Model file for the job. Use its own axes, mm. A direction names the side the tool comes from. Round coordinates to 2 decimals unless told otherwise and drop trailing zeros. Loops run counter-clockwise (first coordinate to the right, second up) from the corner with the lowest first, then second, coordinate; pieces in that order, holes last. Notation, with made-up numbers: (21.25, -7) - (32.25, -7) arc R20 ccw to (32.25, 8) - close; hole circle Ø8 at (-30.5, 56.25). An arc over 180 degrees is marked (long way). Answer as a JSON object with one key per item and string values.
from build123d import *

# Parameters (mm, degrees)
BOX054_W          = 2
BOX054_H          = 2
BOX054_DEPTH      = 2
BOX051_W          = 47.5
BOX051_H          = 17.2
BOX051_DEPTH      = 27
BOX050_W          = 47.5
BOX050_H          = 18.7
BOX050_DEPTH      = 30
BOX053_W          = 10
BOX053_H          = 11.7
BOX053_DEPTH      = 6.2
FILLET001_R       = 3.05
CYLINDER038_R     = 1.7
CYLINDER038_DEPTH = 10
CYLINDER037_R     = 1.7
CYLINDER037_DEPTH = 10
CYLINDER036_R     = 1.7
CYLINDER036_DEPTH = 10
CYLINDER035_R     = 1.7
CYLINDER035_DEPTH = 10
BOX024_W          = 10
BOX024_H          = 10
BOX024_DEPTH      = 10
BOX025_W          = 10
BOX025_H          = 10
BOX025_DEPTH      = 10
CYLINDER023_R     = 4.3
CYLINDER023_DEPTH = 5
CYLINDER019_R     = 1.2
CYLINDER019_DEPTH = 10
BOX013_W          = 4.5
BOX013_H          = 4.5
BOX013_DEPTH      = 10
BOX012_W          = 7.5
BOX012_H          = 7.5
BOX012_DEPTH      = 10
CYLINDER020_R     = 1.2
CYLINDER020_DEPTH = 10
BOX015_W          = 4.5
BOX015_H          = 4.5
BOX015_DEPTH      = 10
BOX014_W          = 7.5
BOX014_H          = 7.5
BOX014_DEPTH      = 10
CYLINDER021_R     = 1.2
CYLINDER021_DEPTH = 10
BOX017_W          = 4.5
BOX017_H          = 4.5
BOX017_DEPTH      = 10
BOX016_W          = 7.5
BOX016_H          = 7.5
BOX016_DEPTH      = 10
CYLINDER022_R     = 1.2
CYLINDER022_DEPTH = 10
BOX019_W          = 4.5
BOX019_H          = 4.5
BOX019_DEPTH      = 10
BOX018_W          = 7.5
BOX018_H          = 7.5
BOX018_DEPTH      = 10
BOX022_W          = 4.5
BOX022_H          = 4.5
BOX022_DEPTH      = 10
BOX021_W          = 4.5
BOX021_H          = 4.5
BOX021_DEPTH      = 10
BOX023_W          = 4.5
BOX023_H          = 4.5
BOX023_DEPTH      = 10
CYLINDER016_R     = 1.2
CYLINDER016_DEPTH = 100
BOX020_W          = 4.5
BOX020_H          = 4.5
BOX020_DEPTH      = 10
CYLINDER015_R     = 1.2
CYLINDER015_DEPTH = 100
BOX010_W          = 124
BOX010_H          = 98
BOX010_DEPTH      = 45
BOX009_W          = 127
BOX009_H          = 101
BOX009_DEPTH      = 45


with BuildPart() as cube054:
    # Box054 → Box054 (new body)
    with BuildSketch(Plane(origin=(77.5, 107.7, 14), x_dir=(1, 0, 0), z_dir=(0, 0, 1))):
        with Locations((1, 1)):
            Rectangle(BOX054_W, BOX054_H)
    extrude(amount=BOX054_DEPTH)


with BuildPart() as cube051:
    # Box051 → Box051 (new body)
    with BuildSketch(Plane(origin=(-1.5, 0, 60), x_dir=(1, 0, 0), z_dir=(0, 0, 1))):
        with Locations((23.75, 8.6)):
            Rectangle(BOX051_W, BOX051_H)
    extrude(amount=BOX051_DEPTH)


with BuildPart() as batteryholder:
    # Box050 → Box050 (new body)
    with BuildSketch(Plane.XY.offset(58.5)):
        with Locations((23.75, 9.35)):
            Rectangle(BOX050_W, BOX050_H)
    extrude(amount=BOX050_DEPTH)

    # Cut062: cut Cube051
    add(cube051.part, mode=Mode.SUBTRACT)


with BuildPart() as batteryholder_1:
    # Cut062 placement: moved
    add(batteryholder.part.moved(Location((77.5, 91, -58.5))))

    # Fusion004: union Cube054
    add(cube054.part)


with BuildPart() as fillet001:
    # Box053 → Box053 (new body)
    with BuildSketch(Plane(origin=(0, -50, 10.3), x_dir=(1, 0, 0), z_dir=(0, 0, 1))):
        with Locations((5, 5.85)):
            Rectangle(BOX053_W, BOX053_H)
    extrude(amount=BOX053_DEPTH)

    # Fillet001
    fillet001_edges = [fillet001.edges().sort_by_distance(p)[0] for p in [
        (5, -50, 10.3),
        (5, -50, 16.5),
        (5, -38.3, 10.3),
        (5, -38.3, 16.5),
    ]]
    fillet(fillet001_edges, radius=FILLET001_R)


with BuildPart() as fillet001_1:
    # Fillet001 placement: moved
    add(fillet001.part.moved(Location((-5, 104, 10))))


with BuildPart() as cylinder038:
    # Cylinder038 → Cylinder038 (new body)
    with BuildSketch(Plane(origin=(126.15, 53.74, 41), x_dir=(0, 0, 1), z_dir=(-1, 0, 0))):
        Circle(CYLINDER038_R)
    extrude(amount=CYLINDER038_DEPTH)


with BuildPart() as cylinder037:
    # Cylinder037 → Cylinder037 (new body)
    with BuildSketch(Plane(origin=(56.29, -11.48, 41), x_dir=(0, 0, 1), z_dir=(0, 1, 0))):
        Circle(CYLINDER037_R)
    extrude(amount=CYLINDER037_DEPTH)


with BuildPart() as cylinder036:
    # Cylinder036 → Cylinder036 (new body)
    with BuildSketch(Plane(origin=(60.26, 82.82, 41), x_dir=(0, 0, 1), z_dir=(0, 1, 0))):
        Circle(CYLINDER036_R)
    extrude(amount=CYLINDER036_DEPTH)


with BuildPart() as cylinder035:
    # Cylinder035 → Cylinder035 (new body)
    with BuildSketch(Plane(origin=(6.21, 35.56, 41), x_dir=(0, 0, 1), z_dir=(-1, 0, 0))):
        Circle(CYLINDER035_R)
    extrude(amount=CYLINDER035_DEPTH)


with BuildPart() as cube024:
    # Box024 → Box024 (new body)
    with BuildSketch(Plane(origin=(53.5, -105, 4), x_dir=(1, 0, 0), z_dir=(0, 0, 1))):
        with Locations((5, 5)):
            Rectangle(BOX024_W, BOX024_H)
    extrude(amount=BOX024_DEPTH)


with BuildPart() as cube025:
    # Box025 → Box025 (new body)
    with BuildSketch(Plane(origin=(36.5, -105, 4), x_dir=(1, 0, 0), z_dir=(0, 0, 1))):
        with Locations((5, 5)):
            Rectangle(BOX025_W, BOX025_H)
    extrude(amount=BOX025_DEPTH)


with BuildPart() as cut034:
    # Cylinder023 → Cylinder023 (new body)
    with BuildSketch(Plane(origin=(50, -100, 9), x_dir=(1, 0, 0), z_dir=(0, -1, 0))):
        Circle(CYLINDER023_R)
    extrude(amount=CYLINDER023_DEPTH)

    # Cut033: cut Cube025
    add(cube025.part, mode=Mode.SUBTRACT)

    # Cut034: cut Cube024
    add(cube024.part, mode=Mode.SUBTRACT)


with BuildPart() as cut034_1:
    # Cut034 placement: moved
    add(cut034.part.moved(Location((-15, 193, 1))))


with BuildPart() as cylinder019:
    # Cylinder019 → Cylinder019 (new body)
    with BuildSketch(Plane(origin=(7.5, 16.5, 105), x_dir=(1, 0, 0), z_dir=(0, 0, 1))):
        Circle(CYLINDER019_R)
    extrude(amount=CYLINDER019_DEPTH)


with BuildPart() as cube013:
    # Box013 → Box013 (new body)
    with BuildSketch(Plane(origin=(5.25, 14.25, 98.5), x_dir=(1, 0, 0), z_dir=(0, 0, 1))):
        with Locations((2.25, 2.25)):
            Rectangle(BOX013_W, BOX013_H)
    extrude(amount=BOX013_DEPTH)


with BuildPart() as cut008:
    # Box012 → Box012 (new body)
    with BuildSketch(Plane(origin=(3.75, 12.75, 100), x_dir=(1, 0, 0), z_dir=(0, 0, 1))):
        with Locations((3.75, 3.75)):
            Rectangle(BOX012_W, BOX012_H)
    extrude(amount=BOX012_DEPTH)

    # Cut007: cut Cube013
    add(cube013.part, mode=Mode.SUBTRACT)

    # Cut008: cut Cylinder019
    add(cylinder019.part, mode=Mode.SUBTRACT)


with BuildPart() as cut008_1:
    # Cut008 placement: moved
    add(cut008.part.moved(Location((0, 0, -100))))


with BuildPart() as cylinder020:
    # Cylinder020 → Cylinder020 (new body)
    with BuildSketch(Plane(origin=(7.5, 16.5, 105), x_dir=(1, 0, 0), z_dir=(0, 0, 1))):
        Circle(CYLINDER020_R)
    extrude(amount=CYLINDER020_DEPTH)


with BuildPart() as cube015:
    # Box015 → Box015 (new body)
    with BuildSketch(Plane(origin=(5.25, 14.25, 98.5), x_dir=(1, 0, 0), z_dir=(0, 0, 1))):
        with Locations((2.25, 2.25)):
            Rectangle(BOX015_W, BOX015_H)
    extrude(amount=BOX015_DEPTH)


with BuildPart() as cut010:
    # Box014 → Box014 (new body)
    with BuildSketch(Plane(origin=(3.75, 12.75, 100), x_dir=(1, 0, 0), z_dir=(0, 0, 1))):
        with Locations((3.75, 3.75)):
            Rectangle(BOX014_W, BOX014_H)
    extrude(amount=BOX014_DEPTH)

    # Cut011: cut Cube015
    add(cube015.part, mode=Mode.SUBTRACT)

    # Cut010: cut Cylinder020
    add(cylinder020.part, mode=Mode.SUBTRACT)


with BuildPart() as cut010_1:
    # Cut010 placement: moved
    add(cut010.part.moved(Location((85, 0, -100))))


with BuildPart() as cylinder021:
    # Cylinder021 → Cylinder021 (new body)
    with BuildSketch(Plane(origin=(7.5, 16.5, 105), x_dir=(1, 0, 0), z_dir=(0, 0, 1))):
        Circle(CYLINDER021_R)
    extrude(amount=CYLINDER021_DEPTH)


with BuildPart() as cube017:
    # Box017 → Box017 (new body)
    with BuildSketch(Plane(origin=(5.25, 14.25, 98.5), x_dir=(1, 0, 0), z_dir=(0, 0, 1))):
        with Locations((2.25, 2.25)):
            Rectangle(BOX017_W, BOX017_H)
    extrude(amount=BOX017_DEPTH)


with BuildPart() as cut013:
    # Box016 → Box016 (new body)
    with BuildSketch(Plane(origin=(3.75, 12.75, 100), x_dir=(1, 0, 0), z_dir=(0, 0, 1))):
        with Locations((3.75, 3.75)):
            Rectangle(BOX016_W, BOX016_H)
    extrude(amount=BOX016_DEPTH)

    # Cut012: cut Cube017
    add(cube017.part, mode=Mode.SUBTRACT)

    # Cut013: cut Cylinder021
    add(cylinder021.part, mode=Mode.SUBTRACT)


with BuildPart() as cut013_1:
    # Cut013 placement: moved
    add(cut013.part.moved(Location((85, 65, -100))))


with BuildPart() as cylinder022:
    # Cylinder022 → Cylinder022 (new body)
    with BuildSketch(Plane(origin=(7.5, 16.5, 105), x_dir=(1, 0, 0), z_dir=(0, 0, 1))):
        Circle(CYLINDER022_R)
    extrude(amount=CYLINDER022_DEPTH)


with BuildPart() as cube019:
    # Box019 → Box019 (new body)
    with BuildSketch(Plane(origin=(5.25, 14.25, 98.5), x_dir=(1, 0, 0), z_dir=(0, 0, 1))):
        with Locations((2.25, 2.25)):
            Rectangle(BOX019_W, BOX019_H)
    extrude(amount=BOX019_DEPTH)


with BuildPart() as cut014:
    # Box018 → Box018 (new body)
    with BuildSketch(Plane(origin=(3.75, 12.75, 100), x_dir=(1, 0, 0), z_dir=(0, 0, 1))):
        with Locations((3.75, 3.75)):
            Rectangle(BOX018_W, BOX018_H)
    extrude(amount=BOX018_DEPTH)

    # Cut015: cut Cube019
    add(cube019.part, mode=Mode.SUBTRACT)

    # Cut014: cut Cylinder022
    add(cylinder022.part, mode=Mode.SUBTRACT)


with BuildPart() as cut014_1:
    # Cut014 placement: moved
    add(cut014.part.moved(Location((0, 65, -100))))


with BuildPart() as cube022:
    # Box022 → Box022 (new body)
    with BuildSketch(Plane(origin=(90.25, 79.25, -2), x_dir=(1, 0, 0), z_dir=(0, 0, 1))):
        with Locations((2.25, 2.25)):
            Rectangle(BOX022_W, BOX022_H)
    extrude(amount=BOX022_DEPTH)


with BuildPart() as cube021:
    # Box021 → Box021 (new body)
    with BuildSketch(Plane(origin=(5.25, 79.25, -2), x_dir=(1, 0, 0), z_dir=(0, 0, 1))):
        with Locations((2.25, 2.25)):
            Rectangle(BOX021_W, BOX021_H)
    extrude(amount=BOX021_DEPTH)


with BuildPart() as cube023:
    # Box023 → Box023 (new body)
    with BuildSketch(Plane(origin=(90.25, 14.25, -2), x_dir=(1, 0, 0), z_dir=(0, 0, 1))):
        with Locations((2.25, 2.25)):
            Rectangle(BOX023_W, BOX023_H)
    extrude(amount=BOX023_DEPTH)


with BuildPart() as cylinder016:
    # Cylinder016 → Cylinder016 (new body)
    with BuildSketch(Plane(origin=(92.5, 16.5, -25), x_dir=(1, 0, 0), z_dir=(0, 0, 1))):
        Circle(CYLINDER016_R)
    extrude(amount=CYLINDER016_DEPTH)


with BuildPart() as cube020:
    # Box020 → Box020 (new body)
    with BuildSketch(Plane(origin=(5.25, 14.25, -2), x_dir=(1, 0, 0), z_dir=(0, 0, 1))):
        with Locations((2.25, 2.25)):
            Rectangle(BOX020_W, BOX020_H)
    extrude(amount=BOX020_DEPTH)


with BuildPart() as cylinder015:
    # Cylinder015 → Cylinder015 (new body)
    with BuildSketch(Plane(origin=(7.5, 16.5, -25), x_dir=(1, 0, 0), z_dir=(0, 0, 1))):
        Circle(CYLINDER015_R)
    extrude(amount=CYLINDER015_DEPTH)


with BuildPart() as cube010:
    # Box010 → Box010 (new body)
    with BuildSketch(Plane(origin=(-0.5, -8.5, 1.5), x_dir=(1, 0, 0), z_dir=(0, 0, 1))):
        with Locations((62, 49)):
            Rectangle(BOX010_W, BOX010_H)
    extrude(amount=BOX010_DEPTH)


with BuildPart() as controlbox:
    # Box009 → Box009 (new body)
    with BuildSketch(Plane(origin=(-2, -10, 0), x_dir=(1, 0, 0), z_dir=(0, 0, 1))):
        with Locations((63.5, 50.5)):
            Rectangle(BOX009_W, BOX009_H)
    extrude(amount=BOX009_DEPTH)

    # Cut006: cut Cube010
    add(cube010.part, mode=Mode.SUBTRACT)

    # Cut009: cut Cylinder015
    add(cylinder015.part, mode=Mode.SUBTRACT)

    # Cut016: cut Cube020
    add(cube020.part, mode=Mode.SUBTRACT)

    # Cut017: cut Cylinder016
    add(cylinder016.part, mode=Mode.SUBTRACT)

    # Cut018: cut Cube023
    add(cube023.part, mode=Mode.SUBTRACT)

    # Cut019: cut Cube021
    add(cube021.part, mode=Mode.SUBTRACT)

    # Cut020: cut Cube022
    add(cube022.part, mode=Mode.SUBTRACT)

    # Connect: union Cut014
    add(cut014_1.part)

    # Connect001: union Cut013
    add(cut013_1.part)

    # Connect002: union Cut010
    add(cut010_1.part)

    # Connect003: union Cut008
    add(cut008_1.part)

    # Cut043: cut Cut034
    add(cut034_1.part, mode=Mode.SUBTRACT)

    # Cut058: cut Cylinder035
    add(cylinder035.part, mode=Mode.SUBTRACT)

    # Cut059: cut Cylinder036
    add(cylinder036.part, mode=Mode.SUBTRACT)

    # Cut060: cut Cylinder037
    add(cylinder037.part, mode=Mode.SUBTRACT)

    # Cut061: cut Cylinder038
    add(cylinder038.part, mode=Mode.SUBTRACT)

    # Cut064: cut Fillet001
    add(fillet001_1.part, mode=Mode.SUBTRACT)

    # Fusion006: union BatteryHolder
    add(batteryholder_1.part)


with BuildPart() as controlbox_1:
    # Fusion006 placement: moved
    add(controlbox.part.moved(Location((0, -79, 0))))


solid = controlbox_1.part
1) Tool access for faces 1 (the flat face through (61, -89, 22)), 2 (the flat face through (7, -1.25, 6)), 3 (the flat face through (92, -60.25, 4)), 4 (the flat face through (61, 12, 22)): list every direction of +Z, -Z, +X, -X, +Y, -Y with a clear straight run to the whole face (end or side of a thin tool).
Values follow:
{"face 1": "+Z, -Z, +X, -X, -Y", "face 2": "+Z", "face 3": "-Z", "face 4": "-X"}
2) Slice it at D-D on y = -70. List the corners of the cut face in (x, z).
Values follow:
{"outline": "(-2, 0) - (125, 0) - (125, 45) - (123.5, 45) - (123.5, 1.5) - (-0.5, 1.5) - (-0.5, 45) - (-2, 45) - close"}
3) Slice it at A-A on y = -43.44. List the corners of the cut face in (x, z).
Values follow:
{"outline": "(-2, 0) - (125, 0) - (125, 45) - (123.5, 45) - (123.5, 1.5) - (-0.5, 1.5) - (-0.5, 39.3) - (-2, 39.3) - close; (-2, 42.7) - (-0.5, 42.7) - (-0.5, 45) - (-2, 45) - close"}
4) Probe probe 1 along Y at (x, z) = (7.5, 8.9); probe 2 along X at (y, z) = (2.5, 9.4); probe 3 along X at (y, z) = (11.4, 41). List the from-to ranges inside material, lowest first.
Values follow:
{"probe 1": "-89 to -87.5, -66.25 to -63.7, -61.3 to -58.75, -1.25 to 1.3, 3.7 to 6.25, 10.5 to 12", "probe 2": "-2 to -0.5, 3.75 to 6.3, 8.7 to 11.25, 88.75 to 91.3, 93.7 to 96.25, 123.5 to 125", "probe 3": "-2 to 58.56, 61.96 to 125"}
5) Drop flat-ended pins along their axis: P1, Ø4, axis at x = 92, y = -64, coming from the +Z side; P2, Ø8, axis at x = 45.5, y = -32.5, coming from the +Z side; P3, Ø2, axis at x = 7.5, y = 2.5, coming from the +Z side. Give the stop position or say it passes through.
Values follow:
{"P1": "z = 10", "P2": "z = 1.5", "P3": "through"}
6) Slice it at B-B on z = 37. List the corners of the cut face in (x, y).
Values follow:
{"outline": "(-2, -89) - (125, -89) - (125, 12) - (-2, 12) - close; hole (-0.5, -87.5) - (123.5, -87.5) - (123.5, 10.5) - (-0.5, 10.5) - close"}
7) Slice it at C-C on x = 56.29. List the corners of the cut face in (y, z), then the cut area to 3 significant figures.
Values follow:
{"outline": "(-89, 0) - (12, 0) - (12, 45) - (10.5, 45) - (10.5, 1.5) - (-87.5, 1.5) - (-87.5, 39.3) - (-89, 39.3) - close; (-89, 42.7) - (-87.5, 42.7) - (-87.5, 45) - (-89, 45) - close", "area": "277 mm²"}
8) Two-plate mould, pull along Z, no slides. Class faces 5 (the cylindrical face through (-1.24, -24.13, 21.217)), 6 (the cylindrical face through (-1.24, -42.29, 39.75)), 7 (the flat face through (8.5, 1.5, 8.5)), 8 (the flat face through (9.75, -63, 4)): pulls with the +Z half, pulls with the -Z half, needs draft (parallel to the pull), parting line crosses it, or undercut.
Values follow:
{"face 5": "undercut", "face 6": "undercut", "face 7": "pulls with the -Z half", "face 8": "needs draft"}
